Source: CAD feature listing. Evaluate the final solid. Frame: model axes, mm. Give positions to 0.01 mm unless a question says otherwise; leave off trailing zeros. Return JSON: item names as keys, results as strings.
from build123d import *

# Parameters (mm, degrees)
SKETCH1_R               = 2.6035
BOSS_EXTRUDE1_DEPTH     = 609.6
SKETCH2_W               = 52.583844564
SKETCH2_H               = 999.926982924
CUT_EXTRUDE1_DEPTH      = 21.082
CUT_EXTRUDE1_DEPTH_BACK = 22.352


with BuildPart() as part:
    # Sketch1 → Boss-Extrude1 (new body, symmetric)
    with BuildSketch(Plane.XY):
        with BuildLine():
            Line((-7.179650497, -8.645192506), (-3.952270251, -5.423690499))
            ThreePointArc((-3.952270251, -5.423690499), (-2.922936451, -4.736929036), (-1.709253557, -4.4958))
            Line((-1.709253557, -4.4958), (1.709253557, -4.4958))
            ThreePointArc((1.709253557, -4.4958), (2.922936451, -4.736929036), (3.952270251, -5.423690499))
            Line((3.952270251, -5.423690499), (7.179650497, -8.645192506))
            ThreePointArc((7.179650497, -8.645192506), (7.41473083, -9.822813117), (6.416408329, -10.4902))
            Line((6.416408329, -10.4902), (4.287512407, -10.4902))
            ThreePointArc((4.287512407, -10.4902), (3.54574862, -10.79744862), (3.2385, -11.539212407))
            Line((3.2385, -11.539212407), (3.2385, -11.650987593))
            ThreePointArc((3.2385, -11.650987593), (3.54574862, -12.39275138), (4.287512407, -12.7))
            Line((4.287512407, -12.7), (5.317126718, -12.7))
            ThreePointArc((5.317126718, -12.7), (5.825126718, -12.192), (6.333126718, -12.7))
            Line((6.333126718, -12.7), (9.550443118, -12.7))
            ThreePointArc((9.550443118, -12.7), (10.058366869, -12.192000006), (10.566443095, -12.699847501))
            ThreePointArc((10.566443095, -12.699847501), (12.082537762, -12.08250727), (12.699846982, -10.566399977))
            ThreePointArc((12.699846982, -10.566399977), (12.192000006, -10.058323491), (12.7, -9.5504))
            Line((12.7, -9.5504), (12.7, -6.3330836))
            ThreePointArc((12.7, -6.3330836), (12.192, -5.8250836), (12.7, -5.3170836))
            Line((12.7, -5.3170836), (12.7, -4.287469289))
            ThreePointArc((12.7, -4.287469289), (12.39275138, -3.545705502), (11.650987593, -3.238456882))
            Line((11.650987593, -3.238456882), (11.539212407, -3.238456882))
            ThreePointArc((11.539212407, -3.238456882), (10.79744862, -3.545705502), (10.4902, -4.287469289))
            Line((10.4902, -4.287469289), (10.4902, -6.402089023))
            ThreePointArc((10.4902, -6.402089023), (9.856505071, -7.351067942), (8.737131347, -7.129408934))
            Line((8.737131347, -7.129408934), (5.441005833, -3.840816462))
            ThreePointArc((5.441005833, -3.840816462), (4.750877967, -2.809883091), (4.5085, -1.593185507))
            Line((4.5085, -1.593185507), (4.5085, 1.593185507))
            ThreePointArc((4.5085, 1.593185507), (4.750877967, 2.809883091), (5.441005833, 3.840816462))
            Line((5.441005833, 3.840816462), (8.737131347, 7.129408934))
            ThreePointArc((8.737131347, 7.129408934), (9.856505071, 7.351067942), (10.4902, 6.402089023))
            Line((10.4902, 6.402089023), (10.4902, 4.287469289))
            ThreePointArc((10.4902, 4.287469289), (10.79744862, 3.545705502), (11.539212407, 3.238456882))
            Line((11.539212407, 3.238456882), (11.650987593, 3.238456882))
            ThreePointArc((11.650987593, 3.238456882), (12.39275138, 3.545705502), (12.7, 4.287469289))
            Line((12.7, 4.287469289), (12.7, 5.3170836))
            ThreePointArc((12.7, 5.3170836), (12.192, 5.8250836), (12.7, 6.3330836))
            Line((12.7, 6.3330836), (12.7, 9.5504))
            ThreePointArc((12.7, 9.5504), (12.192000006, 10.058323491), (12.699846982, 10.566399977))
            ThreePointArc((12.699846982, 10.566399977), (12.082537762, 12.08250727), (10.566443095, 12.699847501))
            ThreePointArc((10.566443095, 12.699847501), (10.058366869, 12.192000006), (9.550443118, 12.7))
            Line((9.550443118, 12.7), (6.333126718, 12.7))
            ThreePointArc((6.333126718, 12.7), (5.825126718, 12.192), (5.317126718, 12.7))
            Line((5.317126718, 12.7), (4.287512407, 12.7))
            ThreePointArc((4.287512407, 12.7), (3.54574862, 12.39275138), (3.2385, 11.650987593))
            Line((3.2385, 11.650987593), (3.2385, 11.539212407))
            ThreePointArc((3.2385, 11.539212407), (3.54574862, 10.79744862), (4.287512407, 10.4902))
            Line((4.287512407, 10.4902), (6.476788598, 10.4902))
            ThreePointArc((6.476788598, 10.4902), (7.432222385, 9.85140422), (7.207036008, 8.724370562))
            Line((7.207036008, 8.724370562), (3.898272566, 5.423169045))
            ThreePointArc((3.898272566, 5.423169045), (2.869120213, 4.736787962), (1.655778399, 4.4958))
            Line((1.655778399, 4.4958), (-1.655778399, 4.4958))
            ThreePointArc((-1.655778399, 4.4958), (-2.869120213, 4.736787962), (-3.898272566, 5.423169045))
            Line((-3.898272566, 5.423169045), (-7.207036008, 8.724370562))
            ThreePointArc((-7.207036008, 8.724370562), (-7.432222385, 9.85140422), (-6.476788598, 10.4902))
            Line((-6.476788598, 10.4902), (-4.287512407, 10.4902))
            ThreePointArc((-4.287512407, 10.4902), (-3.54574862, 10.79744862), (-3.2385, 11.539212407))
            Line((-3.2385, 11.539212407), (-3.2385, 11.650987593))
            ThreePointArc((-3.2385, 11.650987593), (-3.54574862, 12.39275138), (-4.287512407, 12.7))
            Line((-4.287512407, 12.7), (-5.317126718, 12.7))
            ThreePointArc((-5.317126718, 12.7), (-5.825126718, 12.192), (-6.333126718, 12.7))
            Line((-6.333126718, 12.7), (-9.550443118, 12.7))
            ThreePointArc((-9.550443118, 12.7), (-10.058366869, 12.192000006), (-10.566443095, 12.699847501))
            ThreePointArc((-10.566443095, 12.699847501), (-12.082537762, 12.08250727), (-12.699846982, 10.566399977))
            ThreePointArc((-12.699846982, 10.566399977), (-12.192000006, 10.058323491), (-12.7, 9.5504))
            Line((-12.7, 9.5504), (-12.7, 6.3330836))
            ThreePointArc((-12.7, 6.3330836), (-12.192, 5.8250836), (-12.7, 5.3170836))
            Line((-12.7, 5.3170836), (-12.7, 4.287469289))
            ThreePointArc((-12.7, 4.287469289), (-12.39275138, 3.545705502), (-11.650987593, 3.238456882))
            Line((-11.650987593, 3.238456882), (-11.539212407, 3.238456882))
            ThreePointArc((-11.539212407, 3.238456882), (-10.79744862, 3.545705502), (-10.4902, 4.287469289))
            Line((-10.4902, 4.287469289), (-10.4902, 6.402089023))
            ThreePointArc((-10.4902, 6.402089023), (-9.856505071, 7.351067942), (-8.737131347, 7.129408934))
            Line((-8.737131347, 7.129408934), (-5.441005833, 3.840816462))
            ThreePointArc((-5.441005833, 3.840816462), (-4.750877967, 2.809883091), (-4.5085, 1.593185507))
            Line((-4.5085, 1.593185507), (-4.5085, -1.593185507))
            ThreePointArc((-4.5085, -1.593185507), (-4.750877967, -2.809883091), (-5.441005833, -3.840816462))
            Line((-5.441005833, -3.840816462), (-8.737131347, -7.129408934))
            ThreePointArc((-8.737131347, -7.129408934), (-9.856505071, -7.351067942), (-10.4902, -6.402089023))
            Line((-10.4902, -6.402089023), (-10.4902, -4.287469289))
            ThreePointArc((-10.4902, -4.287469289), (-10.79744862, -3.545705502), (-11.539212407, -3.238456882))
            Line((-11.539212407, -3.238456882), (-11.650987593, -3.238456882))
            ThreePointArc((-11.650987593, -3.238456882), (-12.39275138, -3.545705502), (-12.7, -4.287469289))
            Line((-12.7, -4.287469289), (-12.7, -5.3170836))
            ThreePointArc((-12.7, -5.3170836), (-12.192, -5.8250836), (-12.7, -6.3330836))
            Line((-12.7, -6.3330836), (-12.7, -9.5504))
            ThreePointArc((-12.7, -9.5504), (-12.192000006, -10.058323491), (-12.699846982, -10.566399977))
            ThreePointArc((-12.699846982, -10.566399977), (-12.082537762, -12.08250727), (-10.566443095, -12.699847501))
            ThreePointArc((-10.566443095, -12.699847501), (-10.058366869, -12.192000006), (-9.550443118, -12.7))
            Line((-9.550443118, -12.7), (-6.333126718, -12.7))
            ThreePointArc((-6.333126718, -12.7), (-5.825126718, -12.192), (-5.317126718, -12.7))
            Line((-5.317126718, -12.7), (-4.287512407, -12.7))
            ThreePointArc((-4.287512407, -12.7), (-3.54574862, -12.39275138), (-3.2385, -11.650987593))
            Line((-3.2385, -11.650987593), (-3.2385, -11.539212407))
            ThreePointArc((-3.2385, -11.539212407), (-3.54574862, -10.79744862), (-4.287512407, -10.4902))
            Line((-4.287512407, -10.4902), (-6.416408329, -10.4902))
            ThreePointArc((-6.416408329, -10.4902), (-7.41473083, -9.822813117), (-7.179650497, -8.645192506))
        make_face()
        Circle(SKETCH1_R, mode=Mode.SUBTRACT)
    extrude(amount=BOSS_EXTRUDE1_DEPTH, both=True)

    # Sketch2 → Cut-Extrude1 (cut, two sides)
    with BuildSketch(Plane(origin=(-0.793875106, -0.795693603, 0), x_dir=(0.707915262, -0.706297375, 0), z_dir=(-0.706297375, -0.707915262, 0))) as cut_extrude1_sk:
        with Locations((4.622489738, -115.840698227)):
            Rectangle(SKETCH2_W, SKETCH2_H)
    extrude(amount=CUT_EXTRUDE1_DEPTH, mode=Mode.SUBTRACT)
    extrude(cut_extrude1_sk.sketch, amount=-CUT_EXTRUDE1_DEPTH_BACK, mode=Mode.SUBTRACT)


solid = part.part
1. First-contact query: pin 1 (1.7 mm diameter, centred on x = -0.5, z = 470, fed in from +Y); pin 2 (1 mm diameter, centred on y = 0.5, z = 464, fed in from +X); pin 3 (1.7 mm diameter, centred on x = -0.5, z = 476.5, fed in from -Y). Flat tips, straight axial feed; report the tip coordinate or a pass-through.
Evaluation:
{"pin 1": "stops at y = 4.5", "pin 2": "stops at x = 4.51", "pin 3": "stops at y = -4.5"}
2. Draft query along Y for faces 1 (the face through (3, 0, 609.6)), 2 (the face through (2.483, 0.782, 495.283)). Return one class per face: pulls with the +Y half, pulls with the -Y half, needs draft (parallel to the pull), parting line crosses it, or undercut.
Evaluation:
{"face 1": "needs draft", "face 2": "undercut"}
3. Ray query, probe 1 along Y at (x, z) = (-2, 481.5); probe 2 along Y at (x, z) = (0, 526); probe 3 along Y at (x, z) = (3.5, 400.5). Return the intervals inside material, ascending.
Evaluation:
{"probe 1": "y = -4.51 to -1.67, 1.67 to 4.51", "probe 2": "y = -4.5 to -2.6, 2.6 to 4.5", "probe 3": "y = -12.34 to -10.85, -5.05 to 5.09, 10.85 to 12.34"}
